Input: part model. Units: mm. Frame: model coordinates. A direction names the side the tool comes from. Coordinates: 2 decimals unless noted, no trailing zeros. Write each loop counter-clockwise with the first axis right and the second up, starting at its lowest first coordinate (ties: lowest second). Pieces come first, ordered by that corner, then holes. Notation, with made-up numbers: (-4.5, 30) - (23.5, 30) arc R34 ccw to (23.5, 69) - close; hole circle Ø1 at (68.25, -31). An arc over 180 degrees is marked (long way). Put each result on its own line as item: value. Start each with the question number.
1. Cut plane B-B, the plane y = 6.5. Return loops of the section in (x, z).
2. Access query for faces 4 (the flat face through (0, 5, 2)), 5 (the flat face through (-1, 5, 11.5)), 6 (the flat face through (24, 5, 8)), 7 (the flat face through (23, 5, 11.5)), 8 (the flat face through (23, 5, 4.5)). Directions: +Z, -Z, +X, -X, +Y, -Y. A direction counts if a zero-diameter tool reaches every point of the face in a straight line with its end or side. Return the directions, or none.
3. Line query: line 1 (Z direction, x = -0.5, y = 7); line 2 (X direction, y = 2.5, z = 14.5); line 3 (X direction, y = 4, z = 6.5). Output: solid intervals per line, ascending.
4. Pull-direction query (X, two-part tool) for faces 1 (the flat face through (11, 8, 0)), 2 (the cylindrical face through (10.805, 7.203, 7.888)), 3 (the flat face through (0, 5, 14)); classes: released by +X, released by -X, zero draft, split by the parting line, or undercut.
5. Pin query (flat end, axial travel): pin 1 (2 mm diameter, centred on y = 6, z = 13.5, fed in from -X); pin 2 (3 mm diameter, centred on x = 18, z = 10, fed in from -Y); pin 3 (2 mm diameter, centred on x = 23.5, y = 3, fed in from -Z); pin 4 (3.5 mm diameter, centred on y = 5, z = 13, fed in from +X). Return the tip coordinate at first contact, or that it passes through.
6. Cut plane C-C, the plane z = 6.75. Return loops of the section in (x, y), and give its area (3 significant figures).
7. Cut plane A-A, the plane y = 9.25. Return loops of the section in (x, z), and give its area (3 significant figures).
8. Cut plane D-D, the plane x = 2. Return loops of the section in (y, z).
from build123d import *

# Parameters (mm, degrees)
F1_DEPTH = 16
F2_W     = 10
F2_H     = 7
F3_DEPTH = 2
F4_W     = 10
F4_H     = 7
F5_DEPTH = 2


with BuildPart() as f1:
    # F0 (on Top) → F1 (new body)
    with BuildSketch(Plane.XY):
        with BuildLine():
            Line((0, 10), (0, 0))
            ThreePointArc((0, 0), (11, 7.204168), (22, 0))
            Line((22, 0), (22, 10))
            Line((22, 10), (0, 10))
        make_face()
    extrude(amount=F1_DEPTH)

    # F2 (on face) → F3 (join)
    with BuildSketch(Plane.YZ.offset(22)):
        with Locations((5, 8)):
            Rectangle(F2_W, F2_H)
    extrude(amount=F3_DEPTH)

    # F4 (on face) → F5 (join)
    with BuildSketch(Plane(origin=(0, 0, 0), x_dir=(0, -1, 0), z_dir=(-1, 0, 0))):
        with Locations((-5, 8)):
            Rectangle(F4_W, F4_H)
    extrude(amount=F5_DEPTH)


solid = f1.part
Report:
1. outline: (-2, 4.5) - (0, 4.5) - (0, 0) - (6.95, 0) - (6.95, 16) - (0, 16) - (0, 11.5) - (-2, 11.5) - close; (15.05, 0) - (22, 0) - (22, 4.5) - (24, 4.5) - (24, 11.5) - (22, 11.5) - (22, 16) - (15.05, 16) - close
2. face 4: -Z, -X, +Y, -Y
2. face 5: +Z, -X, +Y, -Y
2. face 6: +Z, -Z, +X, +Y, -Y
2. face 7: +Z, +X, +Y, -Y
2. face 8: -Z, +X, +Y, -Y
3. line 1: z = 4.5 to 11.5
3. line 2: x = 0 to 1.47, 20.53 to 22
3. line 3: x = -2 to 2.84, 19.16 to 24
4. face 1: zero draft
4. face 2: undercut
4. face 3: released by -X
5. pin 1: stops at x = 0
5. pin 2: stops at y = 3.67
5. pin 3: stops at z = 4.5
5. pin 4: stops at x = 24
6. outline: (-2, 0) - (0, 0) arc R12 cw to (22, 0) - (24, 0) - (24, 10) - (-2, 10) - close
6. area: 146 mm^2
7. outline: (-2, 4.5) - (0, 4.5) - (0, 0) - (22, 0) - (22, 4.5) - (24, 4.5) - (24, 11.5) - (22, 11.5) - (22, 16) - (0, 16) - (0, 11.5) - (-2, 11.5) - close
7. area: 380 mm^2
8. outline: (3.14, 0) - (10, 0) - (10, 16) - (3.14, 16) - close
